from build123d import *

# Parameters (mm, degrees)
BOSS_EXTRUDE1_DEPTH  = 5
SKETCH2_W            = 6.5
SKETCH2_H            = 5
CUT_EXTRUDE1_DEPTH   = 74.152238517
FILLET1_R            = 10
M5_CLEARANCE_HOLE1_D = 5.8


with BuildPart() as part:
    # Sketch1 → Boss-Extrude1 (new, symmetric)
    with BuildSketch(Plane.XY):
        Polygon((0, 0), (10, 0), (10, -63), (26.5, -63), (26.5, -48), (21.5, -48), (21.5, -58), (20, -58), (20, -10), (26.5, -10), (26.5, 5), (21.5, 5), (21.5, -5), (20, -5), (20, 10), (0, 10), align=None)
    extrude(amount=BOSS_EXTRUDE1_DEPTH, both=True)

    # Sketch2 → Cut-Extrude1 (cut, through all)
    with BuildSketch(Plane(origin=(0, 5, 0), x_dir=(1, 0, 0), z_dir=(0, 1, 0))):
        with Locations((23.25, -2.5)):
            Rectangle(SKETCH2_W, SKETCH2_H)
    extrude(amount=-CUT_EXTRUDE1_DEPTH, mode=Mode.SUBTRACT)

    # Fillet1
    # the kernel refuses this fillet: 10 mm, written as the material it adds along each edge
    with BuildSketch(Plane(origin=(20, -10, -5), x_dir=(0, -1, 0), z_dir=(0, 0, 1))) as fillet1_piece_1:
        with BuildLine():
            CenterArc((9.367496998, 10), FILLET1_R, 200.487315115, 69.512684885)
            Line((0, 6.5), (-0.18734994, 6.43))
            ThreePointArc((-0.18734994, 6.43), (-0.2, 3.25), (-0.2, 0))
            Line((-0.2, 0), (0, -0.2))
            Line((0, -0.2), (9.367496998, -0.2))
            Line((9.367496998, -0.2), (9.367496998, 0))
        make_face()
    extrude(amount=5)

    # M5 Clearance Hole1 (through all)
    with Locations(Plane(origin=(0, 10, 0), x_dir=(1, 0, 0), z_dir=(0, 1, 0))):
        with Locations((5, 0)):
            Hole(M5_CLEARANCE_HOLE1_D / 2)


solid = part.part
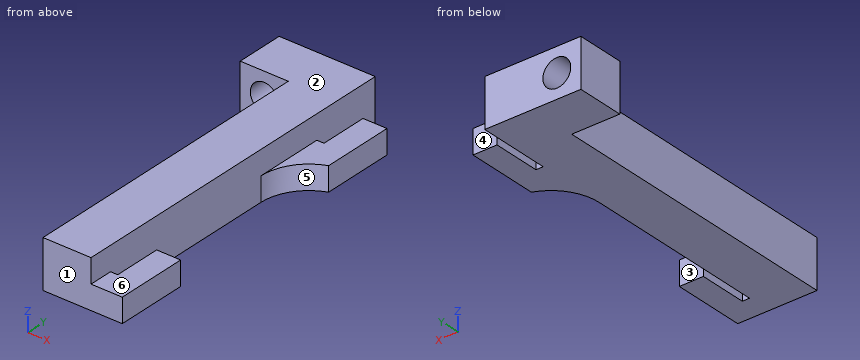
Part model, mm, in its own coordinate system. Face numbers are marked on the shaded views. A direction names the side the tool comes from. Coordinates: 2 decimals unless noted, no trailing zeros. Loops run counter-clockwise (first coordinate to the right, second up) from the corner with the lowest first, then second, coordinate; pieces in that order, holes last. Notation, with made-up numbers: M -0.75,21.25 L 24.25,21.25 A25 ccw 24.25,39.25 Z; hole C 0.25,-3 d9. An arc over 180 degrees is marked long. Use a Markdown table: item, result. Add a question column.
Q1. Cut at C-C (y = -11). Write the cut outline in (x, z), and give its area (3 significant figures).
Q2. Pin check, flat tips, straight feed: P1, Ø5, axis at x = 24.5, y = -58.5, coming from the +Z side; P2, Ø1, axis at y = -23, z = 2, coming from the +X side; P3, Ø1.5, axis at x = 23.5, z = -3.5, coming from the +Y side. Stop position of each tip, or through.
Q3. Which spindle directions (+Z, -Z, +X, -X, +Y, -Y) get a long thin tool onto all of the face, cutting with end or side? Do the marked faces 4, 5 and 6. Say none if no direction does.
Q4. Mould opens along Y. For the marked faces 1, 2 and 3 say: +Y half, -Y half, draft (parallel to the pull), parting line (faces both ways), or undercut.
Q5. Cut at D-D (x = 5). Write the cut outline in (y, z), and give its area (3 significant figures).
Q6. Probe L1, parallel to Z at x = 5, y = 4; L2, parallel to X at y = 1.5, z = 2; L3, parallel to Y at x = 1.75, z = 4. List the from-to ranges inside material, lowest first.
Q7. Cut at B-B (x = 23.75). Write the cut outline in (y, z).
Q8. Cut at A-A (z = -2). Write the cut outline in (x, y).
Worked out:
| question | item | result |
|---|---|---|
| 1 | outline | M 10,-5 L 24.52,-5 L 24.52,0 L 20,0 L 20,5 L 10,5 Z |
| 1 | area | 123 mm2 |
| 2 | P1 | stops at z = 0 |
| 2 | P2 | stops at x = 20 |
| 2 | P3 | stops at y = 5 |
| 3 | face 4 | +Z, -Z, +X, +Y |
| 3 | face 5 | +Z, -Z, +X |
| 3 | face 6 | +Z, +X, +Y, -Y |
| 4 | face 1 | -Y half |
| 4 | face 2 | draft |
| 4 | face 3 | undercut |
| 5 | outline | M 0,-5 L 10,-5 L 10,-2.9 L 0,-2.9 Z; M 0,2.9 L 10,2.9 L 10,5 L 0,5 Z |
| 5 | area | 42.0 mm2 |
| 6 | L1 | z = -5 to -2.9, 2.9 to 5 |
| 6 | L2 | x = 0 to 2.9, 7.1 to 20 |
| 6 | L3 | y = 0 to 10 |
| 7 | outline | M -63,-5 L -48,-5 L -48,0 L -63,0 Z; M -11.56,-5 L 5,-5 L 5,0 L -11.56,0 Z |
| 8 | outline | M 0,0 L 2.9,0 L 2.9,10 L 0,10 Z; M 7.1,0 L 10,0 L 10,-63 L 26.5,-63 L 26.5,-48 L 21.5,-48 L 21.5,-58 L 20,-58 L 20,-19.37 A10 cw 26.5,-10 L 26.5,5 L 21.5,5 L 21.5,-5 L 20,-5 L 20,10 L 7.1,10 Z |
